Here's how the part is built. I have some questions about the finished solid (model axes, mm). A direction names the side the tool comes from. Round coordinates to 2 decimals unless told otherwise and drop trailing zeros. Write each loop counter-clockwise with the first axis right and the second up, starting at its lowest first coordinate (ties: lowest second). Pieces come first, ordered by that corner, then holes. Notation, with made-up numbers: (63.5, 45.5) - (96.5, 45.5) arc R24 cw to (96.5, 72.5) - close; hole circle Ø7 at (-20, 76). An arc over 180 degrees is marked (long way). One line per item, written item: value. Start each with the question number.
Item 1: If I drill on line 1 (Y direction, x = 17, z = 3); line 2 (X direction, y = -18, z = -22); line 3 (Z direction, x = 4, y = 8.5), over which ranges is the centre line in solid material (lowest first)?
Item 2: Thinking about a two-plate mould opening in X: for faces 1 (the face through (-18, 0, 4)), 2 (the face through (6.13, -0.42, -14.78)), 3 (the face through (21.845, 8.979, -0.028)), which applies, released by +X, released by -X, zero draft, split by the parting line, or undercut?
Item 3: Imagine slicing it at D-D, the plane y = 22. Please give me the cut outline in (x, z), then the cut area to 3 significant figures.
Item 4: For faces 4 (the face through (-22, 10, -2)), 5 (the face through (21.6, 8.6, -2)), 6 (the face through (-18, -2.5, 0)), which set-ups out of +Z, -Z, +X, -X, +Y, -Y let a thin tool reach every point of the face, with its end or its side?
Item 5: For P1, Ø3, axis at y = 12, z = 10.5, coming from the +X side; P2, Ø3, axis at x = -24, y = 7.5, coming from the +Z side; P3, Ø4, axis at x = -23, y = 8.5, coming from the -Z side, each with a flat end and sliding along its axis, tell me the tip position at first contact or that it passes through.
Item 6: Imagine slicing it at B-B, the plane z = 0. Count the separate pieces of the cut face and the enclosed holes in it, then the cut area to 3 significant figures.
Item 7: Imagine slicing it at C-C, the plane z = -14. Please give me the cut outline in (x, y), then the cut area to 3 significant figures.
Item 8: Imagine slicing it at A-A, the plane x = 0. Please give me the cut outline in (y, z), then the cut area to 3 significant figures.
```python
from build123d import *

# Parameters (mm, degrees)
CROQUIS1_W              = 40
CROQUIS1_H              = 45
CROQUIS1_R              = 16
SALIENTE_EXTRUIR1_DEPTH = 30
CROQUIS3_W              = 8
CROQUIS3_H              = 5
CORTAR_EXTRUIR1_DEPTH   = 40
CROQUIS4_W              = 6
CROQUIS4_H              = 10
CROQUIS4_R              = 1.25
SALIENTE_EXTRUIR2_DEPTH = 2
REDONDEO1_R             = 5


with BuildPart() as part:
    # Croquis1 → Saliente-Extruir1 (new, symmetric)
    with BuildSketch(Plane(origin=(0, 0, 0), x_dir=(1, 0, 0), z_dir=(0, 1, 0))):
        with Locations((0, 2.5)):
            Rectangle(CROQUIS1_W, CROQUIS1_H)
        with Locations(Location((0, 0, 0), (0, 0, 90))):
            Circle(CROQUIS1_R, mode=Mode.SUBTRACT)
    extrude(amount=SALIENTE_EXTRUIR1_DEPTH, both=True)

    # Croquis3 → Cortar-Extruir1 (cut, symmetric)
    with BuildSketch(Plane(origin=(0, 0, 0), x_dir=(0, 0, -1), z_dir=(1, 0, 0))):
        Rectangle(CROQUIS3_W, CROQUIS3_H)
    extrude(amount=CORTAR_EXTRUIR1_DEPTH, both=True, mode=Mode.SUBTRACT)

    # Croquis4 → Saliente-Extruir2 (add, symmetric)
    # profile 1 of 2: a face of its own
    with BuildSketch(Plane.XY):
        with Locations((-23, 8.5)):
            Rectangle(CROQUIS4_W, CROQUIS4_H)
        with Locations((-23, 8.5)):
            Circle(CROQUIS4_R, mode=Mode.SUBTRACT)
    # profile 2 of 2: a face of its own
    with BuildSketch(Plane.XY):
        with Locations((23, 8.5)):
            Rectangle(CROQUIS4_W, CROQUIS4_H)
        with Locations(Location((23, 8.5, 0), (0, 0, 180))):
            Circle(CROQUIS4_R, mode=Mode.SUBTRACT)
    extrude(amount=SALIENTE_EXTRUIR2_DEPTH, both=True)

    # Redondeo1
    redondeo1_edges = [part.edges().sort_by_distance(p)[0] for p in [
        (26, 3.5, 0),
        (26, 13.5, 0),
        (-26, 3.5, 0),
        (-26, 13.5, 0),
    ]]
    fillet(redondeo1_edges, radius=REDONDEO1_R - 0.0001)  # a hair under: the kernel refuses the full size


solid = part.part
```
Values follow:
1. line 1: y = -30 to -2.5, 2.5 to 30
1. line 2: x = -20 to 20
1. line 3: z = -25 to -15.49, 15.49 to 20
2. face 1: zero draft
2. face 2: undercut
2. face 3: undercut
3. outline: (-20, -25) - (20, -25) - (20, 20) - (-20, 20) - close; hole circle Ø32 at (0, 0)
3. area: 996 mm^2
4. face 4: -Z, -X, +Y, -Y
4. face 5: -Z, +X, +Y, -Y
4. face 6: +X, -X
5. P1: stops at x = 20
5. P2: stops at z = 2
5. P3: stops at z = -2
6. separate pieces: 4
6. enclosed holes: 2
6. area: 529 mm^2
7. outline: (-20, -30) - (-7.75, -30) - (-7.75, 30) - (-20, 30) - close; (7.75, -30) - (20, -30) - (20, 30) - (7.75, 30) - close
7. area: 1,470 mm^2
8. outline: (-30, -25) - (30, -25) - (30, -16) - (-30, -16) - close; (-30, 16) - (30, 16) - (30, 20) - (-30, 20) - close
8. area: 780 mm^2
